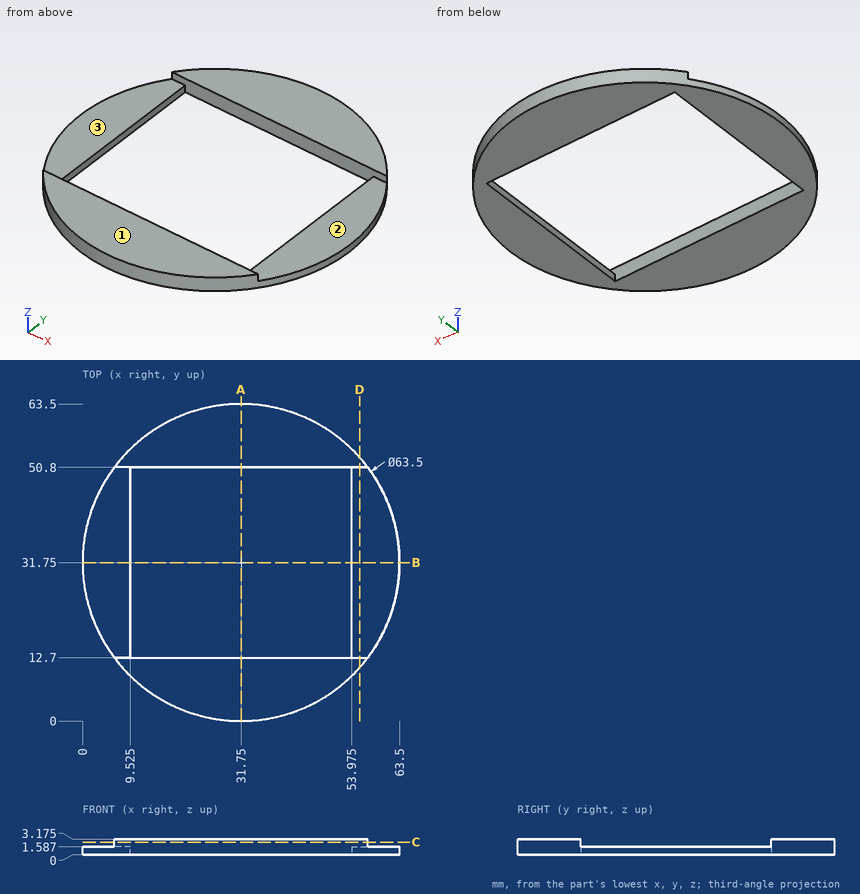
For this review, use the dimensioned drawing (mm, ordinates from the lowest corner) and the shaded views. Round coordinates to 2 decimals unless told otherwise and drop trailing zeros. Write each loop counter-clockwise with the first axis right and the second up, starting at its lowest first coordinate (ties: lowest second). Pieces come first, ordered by that corner, then holes. Notation, with made-up numbers: (80, -40) - (123, -40) arc R11 cw to (123, -31) - close; hole circle Ø1 at (79, -3.5). An arc over 180 degrees is marked (long way). One line per item, written item: value. Start each with the question number.
1. The part is to be moulded in two halves that separate along Y. For the marked faces 1, 2 and 3, say which applies: released by +Y, released by -Y, zero draft, split by the parting line, or undercut.
2. Consider section D-D on x = 55.5. Write out the cut boundary in (y, z) (1 decimal).
3. Consider section C-C on z = 2.55. Write out the cut boundary in (x, y), and give its area (3 significant figures).
4. Consider section B-B on y = 31.75. Write out the cut boundary in (x, z) (1 decimal).
5. To check wall thickness, follow L1, parallel to Z at x = 58.5, y = 17; L2, parallel to X at y = 34.5, z = 1.05 (1 decimal); L3, parallel to Y at x = 23, z = 0.25. State the ranges of each line that lie inside material, in increasing order. Write a range as from..to.
6. Consider section A-A on x = 31.75. Write out the cut boundary in (y, z) (1 decimal).
7. Clearance check with flat-ended pins moving along their axes: P1, Ø5, axis at x = 57.5, y = 37, coming from the +Z side; P2, Ø1, axis at x = 24.5, z = 1.5, coming from the -Y side (1 decimal); P3, Ø1.5, axis at x = 50, z = 2, coming from the -Y side. State where each tip first meets the part, or that it passes through.
Checks:
1. face 1: zero draft
1. face 2: undercut
1. face 3: undercut
2. outline: (10.7, 0) - (52.8, 0) - (52.8, 3.2) - (50.8, 3.2) - (50.8, 1.6) - (12.7, 1.6) - (12.7, 3.2) - (10.7, 3.2) - close
3. outline: (6.35, 12.7) arc R31.75 ccw to (57.15, 12.7) - close; (6.35, 50.8) - (57.15, 50.8) arc R31.75 ccw to start
3. area: 902 mm^2
4. outline: (0, 0) - (9.5, 0) - (9.5, 1.6) - (0, 1.6) - close; (54, 0) - (63.5, 0) - (63.5, 1.6) - (54, 1.6) - close
5. L1: z = 0..1.59
5. L2: x = 0.1..9.5, 54..63.4
5. L3: y = 1.23..12.7, 50.8..62.27
6. outline: (0, 0) - (12.7, 0) - (12.7, 3.2) - (0, 3.2) - close; (50.8, 0) - (63.5, 0) - (63.5, 3.2) - (50.8, 3.2) - close
7. P1: stops at z = 1.59
7. P2: stops at y = 0.7
7. P3: stops at y = 5.26
